Check sheet for the modelled part. Datum: model origin and axes. Units: mm. Give positions to 0.01 mm unless a question says otherwise; leave off trailing zeros. Order: outer loops, then holes, each group sorted by start corner. A loop starts at its lowest first (then second) coordinate and runs counter-clockwise, first axis right, second up.
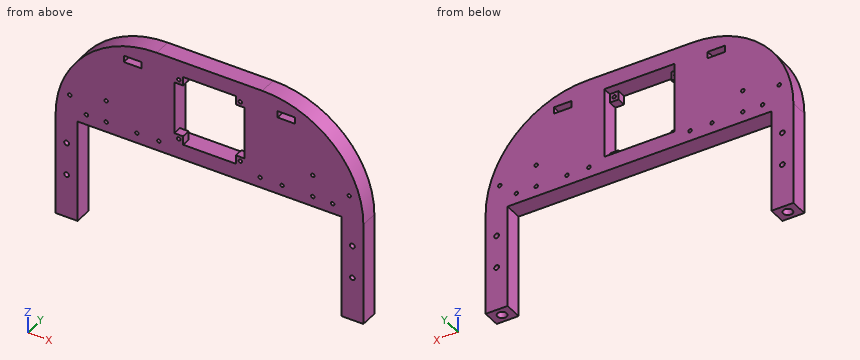
```python
from build123d import *

# Parameters (mm, degrees)
PAD012_DEPTH    = 8
POCKET_DEPTH    = 8.001
SKETCH049_R     = 2.1
HOLE017_DEPTH   = 13.738193
HOLE017_TIPS_R  = 2.1
SKETCH053_W     = 32
SKETCH053_H     = 32
POCKET016_DEPTH = 4
SKETCH054_R     = 0.8
HOLE020_DEPTH   = 25
SKETCH055_W     = 8
SKETCH055_H     = 3
POCKET017_DEPTH = 8.001
SKETCH056_R     = 0.8
HOLE021_DEPTH   = 25
SKETCH058_R     = 1.1
HOLE022_DEPTH   = 25


with BuildPart() as part:
    # Sketch045 → Pad012 (new body)
    with BuildSketch(Plane.XZ):
        with BuildLine():
            Line((-70, 0), (-70, 47))
            ThreePointArc((-24, 93), (-56.526912, 79.526912), (-70, 47))
            Line((-24, 93), (24, 93))
            ThreePointArc((70, 47), (56.526912, 79.526912), (24, 93))
            Line((70, 47), (70, 0))
            Line((70, 0), (60, 0))
            Line((60, 0), (60, 47))
            Line((60, 47), (-60, 47))
            Line((-60, 47), (-60, 0))
            Line((-60, 0), (-70, 0))
        make_face()
    extrude(amount=PAD012_DEPTH)

    # Sketch046 → Pocket (cut, through all)
    with BuildSketch(Plane.XZ):
        Polygon((-12, 82), (-12, 86), (12, 86), (12, 82), (16, 82), (16, 58), (12, 58), (12, 54), (-12, 54), (-12, 58), (-16, 58), (-16, 82), align=None)
    extrude(amount=POCKET_DEPTH, mode=Mode.SUBTRACT)

    # Sketch049 → Hole017 (cut)
    with BuildSketch(Plane(origin=(0, 0, 0), x_dir=(1, 0, 0), z_dir=(0, 0, -1))):
        with Locations((-65, 4)):
            Circle(SKETCH049_R)
        with Locations((65, 4)):
            Circle(SKETCH049_R)
    extrude(amount=-HOLE017_DEPTH, mode=Mode.SUBTRACT)

    # Hole017 tips → Hole017 tip 1 section 0
    with BuildSketch(Plane(origin=(0, 0, 13.738193), x_dir=(1, 0, 0), z_dir=(0, 0, -1)), mode=Mode.PRIVATE) as hole017_tip_1_s0:
        with Locations((-65, 4)):
            Circle(HOLE017_TIPS_R)
    loft([hole017_tip_1_s0.sketch, Vertex(-65, -4, 15)], mode=Mode.SUBTRACT)

    # Hole017 tips → Hole017 tip 2 section 0
    with BuildSketch(Plane(origin=(0, 0, 13.738193), x_dir=(1, 0, 0), z_dir=(0, 0, -1)), mode=Mode.PRIVATE) as hole017_tip_2_s0:
        with Locations((65, 4)):
            Circle(HOLE017_TIPS_R)
    loft([hole017_tip_2_s0.sketch, Vertex(65, -4, 15)], mode=Mode.SUBTRACT)

    # Sketch053 (on Face4 of Hole017) → Pocket016 (cut)
    with BuildSketch(Plane(origin=(0, 0, 0), x_dir=(1, 0, 0), z_dir=(0, 1, 0))):
        with Locations((0, -70)):
            Rectangle(SKETCH053_W, SKETCH053_H)
    extrude(amount=-POCKET016_DEPTH, mode=Mode.SUBTRACT)

    # Sketch054 (on Face4 of Pocket016) → Hole020 (cut)
    with BuildSketch(Plane(origin=(0, 0, 0), x_dir=(1, 0, 0), z_dir=(0, 1, 0))):
        with Locations((-14, -84)):
            Circle(SKETCH054_R)
        with Locations((14, -84)):
            Circle(SKETCH054_R)
        with Locations((-14, -56)):
            Circle(SKETCH054_R)
        with Locations((14, -56)):
            Circle(SKETCH054_R)
    extrude(amount=-HOLE020_DEPTH, mode=Mode.SUBTRACT)

    # Sketch055 (on Face4 of Hole020) → Pocket017 (cut, through all)
    with BuildSketch(Plane(origin=(0, 0, 0), x_dir=(1, 0, 0), z_dir=(0, 1, 0))):
        with Locations((-35, -84.5)):
            Rectangle(SKETCH055_W, SKETCH055_H)
        with Locations((35, -84.5)):
            Rectangle(SKETCH055_W, SKETCH055_H)
    extrude(amount=-POCKET017_DEPTH, mode=Mode.SUBTRACT)

    # Sketch056 (on Face4 of Pocket017) → Hole021 (cut)
    with BuildSketch(Plane(origin=(0, 0, 0), x_dir=(1, 0, 0), z_dir=(0, 1, 0))):
        with Locations((-33, -51.65)):
            Circle(SKETCH056_R)
        with Locations((-23, -51.65)):
            Circle(SKETCH056_R)
        with Locations((23, -51.65)):
            Circle(SKETCH056_R)
        with Locations((33, -51.65)):
            Circle(SKETCH056_R)
        with Locations((-47, -51.65)):
            Circle(SKETCH056_R)
        with Locations((-47, -61.65)):
            Circle(SKETCH056_R)
        with Locations((47, -51.65)):
            Circle(SKETCH056_R)
        with Locations((47, -61.65)):
            Circle(SKETCH056_R)
        with Locations((-63.57, -58.19)):
            Circle(SKETCH056_R)
        with Locations((-56, -51.65)):
            Circle(SKETCH056_R)
        with Locations((56, -51.65)):
            Circle(SKETCH056_R)
        with Locations((63.57, -58.19)):
            Circle(SKETCH056_R)
    extrude(amount=-HOLE021_DEPTH, mode=Mode.SUBTRACT)

    # Sketch058 (on Face4 of Hole021) → Hole022 (cut)
    with BuildSketch(Plane(origin=(0, 0, 0), x_dir=(1, 0, 0), z_dir=(0, 1, 0))):
        with Locations((65, -35)):
            Circle(SKETCH058_R)
        with Locations((65, -20)):
            Circle(SKETCH058_R)
        with Locations((-65, -35)):
            Circle(SKETCH058_R)
        with Locations((-65, -20)):
            Circle(SKETCH058_R)
    extrude(amount=-HOLE022_DEPTH, mode=Mode.SUBTRACT)


with BuildPart() as part_1:
    # Body006021005 placement: moved
    add(part.part.moved(Location((0, -82.56, 8))))


solid = part_1.part
```
Q1. Sectioned sample at A-A, the plane z = 15. Record the cut outline in (x, y), plus the area to 3 significant figures.
Q2. Sectioned sample at C-C, the plane x = 6. Record the cut outline in (y, z).
Q3. Material ranges on line 1 (X direction, y = -82.75, z = 30.5); line 2 (Z direction, x = 6, y = -85.5); line 3 (X direction, y = -88.35, z = 92), recorded low to high.
Q4. Go/stop test with flat-tipped pins: P1, Ø3, axis at y = -89, z = 64.5, coming from the -X side; P2, Ø1.4, axis at x = -63.57, z = 66.19, coming from the -Y side; P3, Ø1.2, axis at y = -87.5, z = 92.5, coming from the -X side; P4, Ø3, axis at x = -31.5, y = -89, coming from the +Z side. Record where each tip stops, or that it passes through.
Q5. Sectioned sample at B-B, the plane z = 49. Record the cut outline in (x, y), plus the area to 3 significant figures.
Filled in:
1. outline: (-70, -90.56) - (-60, -90.56) - (-60, -82.56) - (-70, -82.56) - close; (60, -90.56) - (70, -90.56) - (70, -82.56) - (60, -82.56) - close; hole circle Ø4.2 at (-65, -86.56); hole circle Ø4.2 at (65, -86.56)
1. area: 132 mm2
2. outline: (-90.56, 55) - (-82.56, 55) - (-82.56, 62) - (-90.56, 62) - close; (-90.56, 94) - (-82.56, 94) - (-82.56, 101) - (-90.56, 101) - close
3. line 1: x = -70 to -60, 60 to 70
3. line 2: z = 55 to 62, 94 to 101
3. line 3: x = -51.33 to -39, -31 to -14.8, -13.2 to -12, 12 to 13.2, 14.8 to 31, 39 to 51.33
4. P1: stops at x = -69.3
4. P2: passes through
4. P3: stops at x = -51.47
4. P4: stops at z = 100.61
5. outline: (-70, -90.56) - (-60, -90.56) - (-60, -82.56) - (-70, -82.56) - close; (60, -90.56) - (70, -90.56) - (70, -82.56) - (60, -82.56) - close
5. area: 160 mm2
